The model under review builds one solid part; all positions refer to its coordinate system, in mm. Give positions to 0.01 mm unless a question says otherwise; leave off trailing zeros. Order: outer loops, then holes, each group sorted by start corner. A loop starts at its lowest first (then second) coordinate and runs counter-clockwise, first axis right, second up. Notation, with made-up numbers: (-37.75, -17) - (-11.75, -17) arc R18 cw to (-11.75, 12) - close; hole circle Ø6 at (11.5, 64.5). An arc over 180 degrees is marked (long way). Put each result on its own line as item: value.
Autodesk Inventor part; units mm, degrees
ref_plane "YZ Plane" through (0, 0, 0) normal (1, 0, 0) x (0, 1, 0)
ref_plane "XZ Plane" through (0, 0, 0) normal (0, 1, 0) x (-1, 0, 0)
ref_plane "XY Plane" through (0, 0, 0) normal (0, 0, 1) x (1, 0, 0)
sketch "草圖3" plane through (0, 0, 0) normal (0, 1, 0) x (-1, 0, 0)
  line L0 (0, 0) -> (25, 0)
  line L1 (25, 0) -> (25, -31)
  line L2 (25, -31) -> (0, -31)
  line L3 (0, -31) -> (0, 0)
  circle A0 centre (4, -3.5) radius 1.5
  line L4 (28, -3) -> (25, -3)
  line L5 (25, -3) -> (25, -28)
  line L6 (25, -28) -> (28, -28)
  line L7 (28, -28) -> (28, -3)
  line L8 (28, -14) -> (25, -14)
  line L9 (25, -14) -> (25, -17)
  line L10 (25, -17) -> (28, -17)
  line L11 (28, -17) -> (28, -14)
  line L12 (25, 0) -> (0, 0)
  line L13 (0, 0) -> (0, 15)
  line L14 (0, 15) -> (25, 15)
  line L15 (25, 15) -> (25, 0)
  line L16 (28, 11) -> (25, 11)
  line L17 (25, 11) -> (25, 0)
  line L18 (25, 0) -> (28, 0)
  line L19 (28, 0) -> (28, 11)
  line L20 (0, 15) -> (0, 20)
  line L21 (0, 20) -> (-4, 20)
  line L22 (-4, 20) -> (-4, -31)
  line L23 (-4, -31) -> (-4, -36)
  line L24 (-4, -36) -> (0, -36)
  line L25 (0, -36) -> (0, -31)
  line L26 (17, 15) -> (11, 15)
  line L27 (11, 15) -> (11, 12)
  line L28 (11, 12) -> (17, 12)
  line L29 (17, 12) -> (17, 15)
  line L30 (17, -28) -> (11, -28)
  line L31 (11, -28) -> (11, -31)
  line L32 (11, -31) -> (17, -31)
  line L33 (17, -31) -> (17, -28)
  point P0 (25, -15.5)
  point P1 (25, -15.5)
  point P2 (17, -31)
  dimension "d20" = 25
  dimension "d24" = 27.5
  dimension "d25" = 21
  dimension "d26" = 3
  dimension "d27" = 3
  dimension "d28" = 3
  dimension "d29" = 3
  dimension "d30" = 3
  dimension "d31" = 3
  dimension "d33" = 3
  dimension "d34" = 11
  dimension "d35" = 5
  dimension "d36" = 4
  dimension "d37" = 5
  dimension "d38" = 3
  dimension "d39" = 6
  dimension "d40" = 3
  dimension "d41" = 8
extrude "擠出4" add sketch "草圖3" along normal blind 3 contours L13 L14 L27 L28 L29 L15 L0 | L0 L1 L2 L33 L30 L31 L3 | L3 L25 L24 L23 L22 L21 L20 L13 | L15 L16 L19 L18 | L4 L7 L8 L1 | L10 L7 L6 L1
properties material "MDF Medium Density Fiberboard"
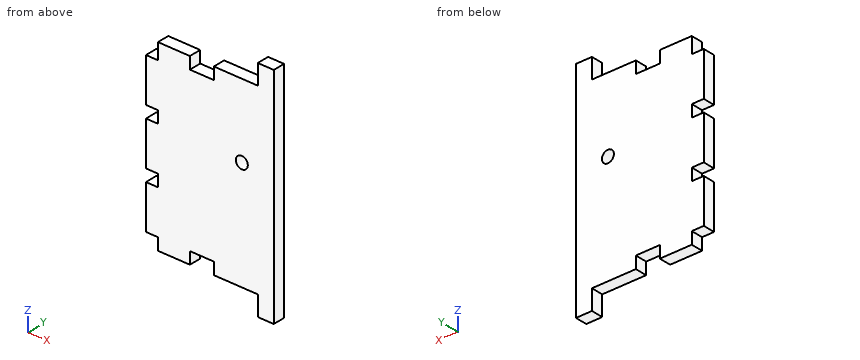
(1) Take a section at A-A, the plane x = -4. Write out the cut boundary in (y, z), then the cut area to 3 significant figures.
The answers:
outline: (0, -31) - (3, -31) - (3, -5) - (0, -5) - close; (0, -2) - (3, -2) - (3, 15) - (0, 15) - close
area: 129 mm^2
(2) Clearance check with flat-ended pins moving along their axes: pin 1 Ø1.5 at (x, y) = (-26, 2) entering from -Z; pin 2 Ø1.5 at (y, z) = (2, -34.5) entering from -X; pin 3 Ø1.5 at (y, z) = (1.5, -1.5) entering from -X. State where each tip first meets the part, or that it passes through.
The answers:
pin 1: z = -28
pin 2: x = 0
pin 3: x = -25
(3) Take a section at D-D, the plane x = -7.5. Write out the cut boundary in (y, z), then the cut area to 3 significant figures.
The answers:
outline: (0, -31) - (3, -31) - (3, 15) - (0, 15) - close
area: 138 mm^2
(4) Wall thickness on L1, parallel to X at y = 2.1, z = -28.5; L2, parallel to Z at x = -4, y = 1.25; L3, parallel to Z at x = -13.5, y = 2.1: over which ranges is each line inside the solid? List them lowest first.
The answers:
L1: -25 to -17, -11 to 4
L2: -31 to -5, -2 to 15
L3: -28 to 12
(5) Take a section at C-C, the plane z = -15. Write out the cut boundary in (x, y), then the cut area to 3 significant figures.
The answers:
outline: (-25, 0) - (4, 0) - (4, 3) - (-25, 3) - close
area: 87.0 mm^2
